Source: CAD feature listing. Evaluate the final solid. Frame: model axes, mm. Face numbers are marked on the shaded views. A direction names the side the tool comes from. Round coordinates to 2 decimals unless told otherwise and drop trailing zeros. Loops run counter-clockwise (first coordinate to the right, second up) from the corner with the lowest first, then second, coordinate; pieces in that order, holes last. Notation, with made-up numbers: M 74,-3 L 78,-3 A7 cw 78,3 Z; hole C 83,1 d6. An arc over 180 degrees is marked long. Answer as a JSON object with one key per item and string values.
Autodesk Inventor part; units mm, degrees
ref_plane "YZ Plane" through (0, 0, 0) normal (1, 0, 0) x (0, 1, 0)
ref_plane "XZ Plane" through (0, 0, 0) normal (0, 1, 0) x (-1, 0, 0)
ref_plane "XY Plane" through (0, 0, 0) normal (0, 0, 1) x (1, 0, 0)
sketch "Sketch1" plane through (0, 0, 0) normal (0, 0, 1) x (1, 0, 0)
  line L0 (17.4112, 0) -> (20.3, 0)
  circle A0 centre (43.66, 15) radius 1.5
  circle A1 centre (-3.96, 4.8) radius 1.5
  line L1 (29.8, -3.5) -> (31.05, -3.5)
  line L2 (31.05, -23.3) -> (28.55, -23.3)
  line L3 (28.55, -23.3) -> (28.55, -3.5)
  line L4 (28.55, -3.5) -> (29.8, -3.5)
  line L5 (29.8, -23.3) -> (29.8, -28.3)
  circle A2 centre (29.8, -28.3) radius 1.5
  line L6 (31.05, -23.3) -> (31.05, -13.9)
  line L7 (31.05, -13.9) -> (33.55, -13.9)
  line L8 (33.55, -13.9) -> (33.55, -12.9)
  line L9 (33.55, -12.9) -> (31.05, -12.9)
  line L10 (31.05, -12.9) -> (31.05, -3.5)
  line L11 (36.55, -14.9) -> (36.55, -28.3)
  line L12 (49.7, 17.8) -> (49.7, 5)
  line L13 (36.55, -13) -> (36.55, -14.9)
  arc A3 (24.55, -28.3) -> (36.55, -28.3) centre (30.55, -28.3) ccw
  line L14 (24.55, -27.924) -> (24.55, -28.3)
  line L15 (5.8588, -8.6221) -> (20.6471, -19.9978)
  circle A4 centre (29.8, 9.9) radius 1.5
  arc A5 (29.8, 14.4) -> (25.3, 9.9) centre (29.8, 9.9) ccw
  line L16 (25.3, 9.9) -> (25.3, 5)
  line L17 (36.55, -13) -> (36.55, -5)
  line L18 (44.7, 0) -> (41.55, 0)
  line L19 (36.3, 14.4) -> (29.8, 14.4)
  arc A6 (36.3, 14.4) -> (39.7, 17.8) centre (36.3, 17.8) ccw
  arc A7 (41.55, 0) -> (36.55, -5) centre (41.55, -5) ccw
  arc A8 (44.7, 0) -> (49.7, 5) centre (44.7, 5) ccw
  arc A9 (20.3, 0) -> (25.3, 5) centre (20.3, 5) ccw
  arc A10 (24.55, -27.924) -> (20.6471, -19.9978) centre (14.55, -27.924) ccw
  line L20 (-3.96, 9.9) -> (-2.2612, 9.9)
  line L21 (-3.96, 9.9) -> (-5, 9.9)
  line L22 (-10, 4.9) -> (-10, 4.7)
  line L23 (11.3141, 2.0738) -> (3.8359, 7.8262)
  arc A11 (11.3141, 2.0738) -> (17.4112, 0) centre (17.4112, 10) ccw
  arc A12 (3.8359, 7.8262) -> (-2.2612, 9.9) centre (-2.2612, -0.1) ccw
  arc A13 (-5, 9.9) -> (-10, 4.9) centre (-5, 4.9) ccw
  arc A14 (-10, 4.7) -> (-5.7001, -0.2507) centre (-5, 4.7) ccw
  line L24 (5.8588, -8.6221) -> (-4.2953, -0.8401)
  arc A15 (-4.2953, -0.8401) -> (-5.7001, -0.2507) centre (-6.1202, -3.2212) ccw
  line L25 (39.7, 17.8) -> (39.7, 17.8)
  line L26 (49.7, 17.8) -> (49.7, 17.8)
  line L27 (44.7, 20.8) -> (46.7, 20.8)
  line L28 (44.7, 20.8) -> (42.7, 20.8)
  arc A16 (42.7, 20.8) -> (39.7, 17.8) centre (42.7, 17.8) ccw
  arc A17 (49.7, 17.8) -> (46.7, 20.8) centre (46.7, 17.8) ccw
  dimension "d13" = 1.25
  dimension "d15" = 2.5
  dimension "d16" = 19.8
  dimension "d17" = 5
  dimension "d25" = 9.4
  dimension "d26" = 2.5
  dimension "d27" = 1
  dimension "d70" = 5
  dimension "d71" = 5
  dimension "d72" = 10
  dimension "d79" = 10
  dimension "d80" = 5
  dimension "d83" = 3
  dimension "d85" = 3
extrude "Extrusion1" add sketch "Sketch1" along normal blind 5
properties part number "braket bawah 2"
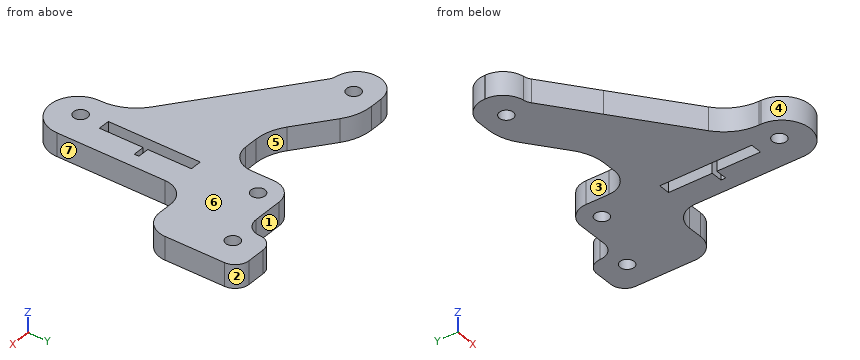
Item 1: Section B-B on z = 2.9. Give the number of separate pieces and of enclosed holes in the cut face, then the cut area to 3 significant figures.
Answer sheet:
{"separate pieces": "1", "enclosed holes": "5", "area": "1,240 mm²"}
Item 2: Line query: probe 1 along X at (y, z) = (3.5, 4); probe 2 along X at (y, z) = (-28.5, 1); probe 3 along Y at (x, z) = (29.8, 3.55). Output: solid intervals per line, ascending. Write a range as from..to.
Answer sheet:
{"probe 1": "x = -9.85..-4.71, -3.21..9.46, 25.07..49.47", "probe 2": "x = 24.55..28.31, 31.29..36.55", "probe 3": "y = -34.25..-29.8, -26.8..-23.3, -3.5..8.4, 11.4..14.4"}
Item 3: Section C-C on x = 0. Return the cut outline in (y, z).
Answer sheet:
{"outline": "M -4.13,0 L 9.64,0 L 9.64,5 L -4.13,5 Z"}
Item 4: Contact query for flat-ended pins moving along their axis: pin 1 Ø2.5 at (x, y) = (43.66, 15) entering from -Z; pin 2 Ø2 at (x, z) = (30.5, 1.5) entering from +Y; pin 3 Ø1.5 at (y, z) = (8.5, 2) entering from -X; pin 4 Ø3 at (x, z) = (34, 1.5) entering from -Y. Output: stop coordinate, or through.
Answer sheet:
{"pin 1": "passes through", "pin 2": "stops at y = 14.4", "pin 3": "stops at x = -9.11", "pin 4": "stops at y = -33.97"}
Item 5: Section A-A on y = -15. Return the cut outline in (x, z).
Answer sheet:
{"outline": "M 14.15,0 L 28.55,0 L 28.55,5 L 14.15,5 Z; M 31.05,0 L 36.55,0 L 36.55,5 L 31.05,5 Z"}
Item 6: Pull-direction query (X, two-part tool) for the marked faces 4, 5, 6 and 7; classes: pulls with the +X half, pulls with the -X half, needs draft (parallel to the pull), parting line crosses it, or undercut.
Answer sheet:
{"face 4": "parting line crosses it", "face 5": "undercut", "face 6": "needs draft", "face 7": "pulls with the +X half"}
Item 7: Access query for the marked faces 1, 2 and 3. Directions: +Z, -Z, +X, -X, +Y, -Y. A direction counts if a zero-diameter tool reaches every point of the face in a straight line with its end or side. Return the directions, or none.
Answer sheet:
{"face 1": "+Z, -Z, -X, +Y", "face 2": "+Z, -Z, +X, +Y", "face 3": "+Z, -Z, +Y"}
